Here's how the part is built. I have some questions about the finished solid (model axes, mm). A direction names the side the tool comes from. Round coordinates to 2 decimals unless told otherwise and drop trailing zeros. Loops run counter-clockwise (first coordinate to the right, second up) from the corner with the lowest first, then second, coordinate; pieces in that order, holes last. Notation, with made-up numbers: (50.5, 9.5) -> (72.5, 9.5) arc R18 ccw to (72.5, 27.5) -> close; hole circle Ø10 at (-31.5, 44.25). An arc over 180 degrees is marked (long way). Use CSV: the item, a comma, the result in double quotes. Start each with the question number.
from build123d import *

# Parameters (mm, degrees)
F4_DEPTH  = 8.9
F6_W      = 6
F6_H      = 8
F7_DEPTH  = 3.7
F8_R      = 0.3
F9_DEPTH  = 3.701
F11_DEPTH = 3


with BuildPart() as f4:
    # F3 (on Right) → F4 (new body)
    with BuildSketch(Plane.YZ):
        Polygon((0, 1.55), (0, 0), (0, -1.55), (16, -1.55), (16, 0), (16, 1.55), align=None)
    extrude(amount=F4_DEPTH)

    # F6 (on offset) → F7 (join)
    with BuildSketch(Plane.XY.offset(1.85)):
        with Locations((4.45, 12)):
            Rectangle(F6_W, F6_H)
    extrude(amount=-F7_DEPTH)

    # F8 (on offset) → F9 (cut, through all)
    with BuildSketch(Plane.XY.offset(1.85)):
        with BuildLine():
            ThreePointArc((1.4, 4), (1.6928932188, 3.2928932188), (2.4, 3))
            Line((2.4, 3), (6.5, 3))
            ThreePointArc((6.5, 3), (7.2071067812, 3.2928932188), (7.5, 4))
            Line((7.5, 4), (7.5, 5.5))
            ThreePointArc((7.5, 5.5), (7.2071067812, 6.2071067812), (6.5, 6.5))
            Line((6.5, 6.5), (2.4, 6.5))
            ThreePointArc((2.4, 6.5), (1.6928932188, 6.2071067812), (1.4, 5.5))
            Line((1.4, 5.5), (1.4, 4))
        make_face()
        with Locations((2.75, 12.65)):
            Circle(F8_R)
        with Locations((6.15, 12.65)):
            Circle(F8_R)
    extrude(amount=-F9_DEPTH, mode=Mode.SUBTRACT)

    # F10 (on face) → F11 (cut, through all)
    with BuildSketch(Plane.XZ):
        with BuildLine():
            Line((5.3, 1.55), (3.6, 1.55))
            Line((3.6, 1.55), (3.6, 0.6982120022))
            ThreePointArc((3.6, 0.6982120022), (4.45, -1.1), (5.3, 0.6982120022))
            Line((5.3, 0.6982120022), (5.3, 1.55))
        make_face()
    extrude(amount=-F11_DEPTH, mode=Mode.SUBTRACT)


solid = f4.part
Q1. I need wall thicknesses on line 1 along Y through (x, z) = (6.15, -0.8); line 2 along X through (y, z) = (1.4, 0); line 3 along Y through (x, z) = (3.5, 1.35). Which ranges of each line are inside material? Lowest first, please.
Q2. If we mould it in two halves opening along Y, with no side actions, what happens to faces 1 (the flat face through (3, 0, 0)), 2 (the cylindrical face through (7.199, 3.285, 0.022)), 3 (the flat face through (8.9, 8, 0))? For each: pulls with the +Y half, pulls with the -Y half, needs draft (parallel to the pull), parting line crosses it, or undercut.
Q3. For faces 4 (the flat face through (0, 8, 0)), 5 (the flat face through (4, 16, 0)), 6 (the flat face through (4.4, 3, -1.4)), 7 (the flat face through (5.3, 1, 1)), 8 (the cylindrical face through (4.4, 1.5, -1.1)), which set-ups out of +Z, -Z, +X, -X, +Y, -Y let a thin tool reach every point of the face, with its end or its side?
Q4. I want a section at A-A, the plane x = 2.75. List the corners of the cut face in (y, z) for me.
Q5. Will these pins go through, and if not, where does the flat tip stop? pin 1 Ø4 at (x, y) = (4, 2.5) entering from -Z; pin 2 Ø1.5 at (x, z) = (3.5, 0) entering from -Y; pin 3 Ø2 at (x, y) = (3.5, 2) entering from +Z.
Q6. I want a section at B-B, the plane y = 4.5. List the corners of the cut face in (x, z) for me.
Q7. I want a section at C-C, the plane y = 12.65. List the corners of the cut face in (x, z) for me, then the cut area to 4 significant figures.
Q8. I want a section at D-D, the plane z = 0. List the corners of the cut face in (x, y) for me, then the cut area to 3 significant figures.
Values found:
1,line 1,"0 to 3, 6.5 to 12.35, 12.95 to 16"
1,line 2,"0 to 3.35, 5.55 to 8.9"
1,line 3,"0 to 3, 6.5 to 16"
2,face 1,"pulls with the -Y half"
2,face 2,"undercut"
2,face 3,"needs draft"
3,face 4,"+Z, -Z, -X, +Y, -Y"
3,face 5,"+Z, -Z, +X, -X, +Y"
3,face 6,"+Z, -Z"
3,face 7,"+Z, -Y"
3,face 8,"-Y"
4,outline,"(0, -1.55) -> (3, -1.55) -> (3, 1.55) -> (0, 1.55) -> close; (6.5, -1.55) -> (8, -1.55) -> (8, -1.85) -> (12.35, -1.85) -> (12.35, 1.85) -> (8, 1.85) -> (8, 1.55) -> (6.5, 1.55) -> close; (12.95, -1.85) -> (16, -1.85) -> (16, 1.85) -> (12.95, 1.85) -> close"
5,pin 1,"z = -1.55"
5,pin 2,"y = 0"
5,pin 3,"z = 1.55"
6,outline,"(0, -1.55) -> (1.4, -1.55) -> (1.4, 1.55) -> (0, 1.55) -> close; (7.5, -1.55) -> (8.9, -1.55) -> (8.9, 1.55) -> (7.5, 1.55) -> close"
7,outline,"(0, -1.55) -> (1.45, -1.55) -> (1.45, -1.85) -> (2.45, -1.85) -> (2.45, 1.85) -> (1.45, 1.85) -> (1.45, 1.55) -> (0, 1.55) -> close; (3.05, -1.85) -> (5.85, -1.85) -> (5.85, 1.85) -> (3.05, 1.85) -> close; (6.45, -1.85) -> (7.45, -1.85) -> (7.45, -1.55) -> (8.9, -1.55) -> (8.9, 1.55) -> (7.45, 1.55) -> (7.45, 1.85) -> (6.45, 1.85) -> close"
7,area,"26.75 mm2"
8,outline,"(0, 0) -> (3.35, 0) -> (3.35, 3) -> (2.4, 3) arc R1 cw to (1.4, 4) -> (1.4, 5.5) arc R1 cw to (2.4, 6.5) -> (6.5, 6.5) arc R1 cw to (7.5, 5.5) -> (7.5, 4) arc R1 cw to (6.5, 3) -> (5.55, 3) -> (5.55, 0) -> (8.9, 0) -> (8.9, 16) -> (0, 16) -> close; hole circle Ø0.6 at (2.75, 12.65); hole circle Ø0.6 at (6.15, 12.65)"
8,area,"115 mm2"
